Check sheet for the modelled part. Datum: model origin and axes. Units: mm. A direction names the side the tool comes from. Round coordinates to 2 decimals unless told otherwise and drop trailing zeros. Loops run counter-clockwise (first coordinate to the right, second up) from the corner with the lowest first, then second, coordinate; pieces in that order, holes last. Notation, with made-up numbers: (-32.75, 20) -> (-12.75, 20) arc R23 ccw to (-12.75, 54) -> close; hole circle Ø1 at (22.25, 80). An arc over 180 degrees is marked (long way). One line per question, with ' | ' between items.
Autodesk Inventor part; units mm, degrees
ref_plane "YZ Plane" through (0, 0, 0) normal (1, 0, 0) x (0, 1, 0)
ref_plane "XZ Plane" through (0, 0, 0) normal (0, 1, 0) x (-1, 0, 0)
ref_plane "XY Plane" through (0, 0, 0) normal (0, 0, 1) x (1, 0, 0)
sketch "Sketch1" plane through (0, 0, 0) normal (0, 1, 0) x (-1, 0, 0)
  line L0 (10.352, 30.898) -> (-9.648, 30.898)
  line L1 (-9.648, 30.898) -> (-9.648, -24.102)
  line L2 (-9.648, -24.102) -> (10.352, -24.102)
  line L3 (10.352, -24.102) -> (10.352, 30.898)
  circle A0 centre (4.852, 26.898) radius 1.75
  circle A1 centre (-3.148, 26.898) radius 1.75
  circle A2 centre (4.852, -20.102) radius 1.75
  circle A3 centre (-3.148, -20.102) radius 1.75
  point P0 (0, 0)
  dimension "d0" = 55
  dimension "d1" = 20
  dimension "d2" = 3.5
  dimension "d3" = 3.5
  dimension "d4" = 3.5
  dimension "d5" = 3.5
  dimension "d6" = 4
  dimension "d7" = 4
  dimension "d8" = 4
  dimension "d9" = 4
  dimension "d10" = 5.5
  dimension "d11" = 8
  dimension "d12" = 5.5
  dimension "d13" = 8
extrude "Extrusion1" add sketch "Sketch1" along normal blind 2
sketch "Sketch2" plane through (0, 2, 0) normal (0, 1, 0) x (1, 0, 0)
  line L0 (9.648, -30.898) -> (9.648, 24.102)
  line L1 (9.648, -20.398) -> (7.648, -20.398)
  line L2 (7.648, -20.398) -> (7.648, 13.602)
  line L3 (7.648, 13.602) -> (9.648, 13.602)
  line L4 (9.648, 13.602) -> (9.648, -20.398)
  line L5 (-10.352, -30.898) -> (9.648, -30.898)
  line L6 (9.648, 24.102) -> (-10.352, 24.102)
  point P0 (0, 0)
  dimension "d16" = 2
  dimension "d17" = 34
  dimension "d18" = 10.5
  dimension "d19" = 10.5
extrude "Extrusion2" add sketch "Sketch2" along normal blind 5
fillet "Fillet1" radius 2 2 edges at (-10.352, 1, 30.898) (-10.352, 1, -24.102)
properties part number "SwitchMountTop"
(1) Set-up check for faces 4 (the face through (7.648, 4, 4)), 5 (the face through (1, 1, -24.102)), 6 (the face through (9, 4, 20.398)): record each of +Z, -Z, +X, -X, +Y, -Y from which the full face is reachable in a straight line by a thin tool's end or side.
Answer:
face 4: +Z, -Z, -X, +Y | face 5: -Z, +X, -X, +Y, -Y | face 6: +Z, +X, -X, +Y
(2) Mould release check, pull along Z, two halves, no side actions. Record for faces 1 (the face through (9, 4, -13.602)), 2 (the face through (-9.78, 1.01, 30.3)), 3 (the face through (-4.473, 0.986, 28.606)): +Z half, -Z half, draft (parallel to the pull), parting line (faces both ways), or undercut.
Answer:
face 1: -Z half | face 2: +Z half | face 3: undercut
(3) Sectioned sample at D-D, the plane y = 6. Record the cut outline in (x, z), and give its area (3 significant figures).
Answer:
outline: (7.65, -13.6) -> (9.65, -13.6) -> (9.65, 20.4) -> (7.65, 20.4) -> close | area: 68.0 mm2
(4) Sectioned sample at C-C, the plane z = -17. Record the cut outline in (x, y), and give its area (3 significant figures).
Answer:
outline: (-10.35, 0) -> (9.65, 0) -> (9.65, 2) -> (-10.35, 2) -> close | area: 40.0 mm2
(5) Go/stop test with flat-tipped pins: pin 1 (12 mm diameter, centred on x = 6.5, z = 15, fed in from -Y); pin 2 (1.6 mm diameter, centred on x = 8.5, y = 4.5, fed in from +Z); pin 3 (1.5 mm diameter, centred on y = 4, z = -10, fed in from -X); pin 4 (2 mm diameter, centred on x = 8.5, y = 3.5, fed in from -Z). Record where each tip stops, or that it passes through.
Answer:
pin 1: stops at y = 0 | pin 2: stops at z = 20.4 | pin 3: stops at x = 7.65 | pin 4: stops at z = -13.6
(6) Sectioned sample at B-B, the plane y = 1.25. Record the cut outline in (x, z), and give its area (3 significant figures).
Answer:
outline: (-10.35, -22.1) arc R2 ccw to (-8.35, -24.1) -> (9.65, -24.1) -> (9.65, 30.9) -> (-8.35, 30.9) arc R2 ccw to (-10.35, 28.9) -> close; hole circle Ø3.5 at (-4.85, -20.1); hole circle Ø3.5 at (-4.85, 26.9); hole circle Ø3.5 at (3.15, -20.1); hole circle Ø3.5 at (3.15, 26.9) | area: 1,060 mm2
(7) Sectioned sample at A-A, the plane x = -4. Record the cut outline in (y, z).
Answer:
outline: (0, -24.1) -> (2, -24.1) -> (2, -21.63) -> (0, -21.63) -> close; (0, -18.57) -> (2, -18.57) -> (2, 25.37) -> (0, 25.37) -> close; (0, 28.43) -> (2, 28.43) -> (2, 30.9) -> (0, 30.9) -> close
(8) Scan lines: probe 1 along Z at (x, y) = (-6.25, 1); probe 2 along Y at (x, z) = (-9, 10); probe 3 along X at (y, z) = (4.5, -4). Record each from-to range of solid material in increasing order.
Answer:
probe 1: z = -24.1 to -21.15, -19.05 to 25.85, 27.95 to 30.9 | probe 2: y = 0 to 2 | probe 3: x = 7.65 to 9.65
